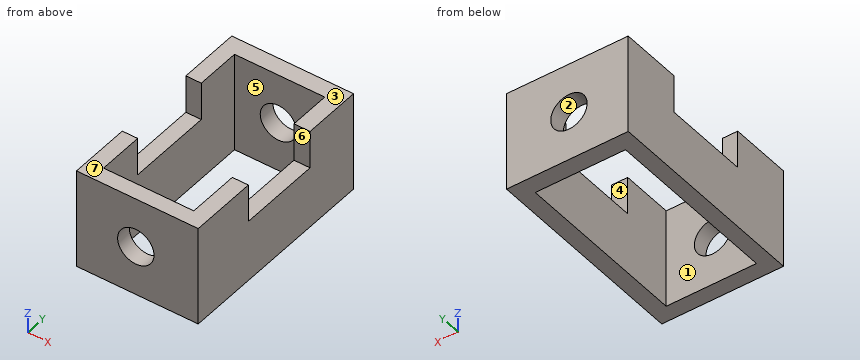
```python
from build123d import *

# Parameters (mm, degrees)
F0_W     = 62.4194853008
F0_H     = 107.7802851796
F0_W_2   = 46.2748277932
F0_H_2   = 90.9063592553
F1_DEPTH = 51.308
F2_W     = 8.2461107522
F2_H     = 42.7914112806
F2_W_2   = 7.8985467553
F2_H_2   = 44.1445242614
F3_DEPTH = 19.558
F4_R     = 9.3280185705
F5_DEPTH = 152.4


with BuildPart() as f1:
    # F0 (on Top) → F1 (new body)
    with BuildSketch(Plane.XY):
        with Locations((-31.2097426504, -8.8457427919)):
            Rectangle(F0_W, F0_H)
        with Locations((-31.3835246488, -9.2003643513)):
            Rectangle(F0_W_2, F0_H_2, mode=Mode.SUBTRACT)
    extrude(amount=F1_DEPTH)

    # F2 (on face) → F3 (cut)
    with BuildSketch(Plane.XY.offset(51.308)):
        with Locations((-4.1230553761, -6.5223816782)):
            Rectangle(F2_W, F2_H)
        with Locations((-58.4702119231, -8.8798655197)):
            Rectangle(F2_W_2, F2_H_2)
    extrude(amount=-F3_DEPTH, mode=Mode.SUBTRACT)

    # F4 (on face) → F5 (cut)
    with BuildSketch(Plane(origin=(0, 45.0443997979, 0), x_dir=(-1, 0, 0), z_dir=(0, 1, 0))):
        with Locations((32.0103727281, 25.654)):
            Circle(F4_R)
    extrude(amount=-F5_DEPTH, mode=Mode.SUBTRACT)


solid = f1.part
```
Can you work these out from the model? Positions are in its coordinate system, mm. Face numbers are marked on the shaded views. A direction names the side the tool comes from. Coordinates: 2 decimals unless noted, no trailing zeros. Loops run counter-clockwise (first coordinate to the right, second up) from the corner with the lowest first, then second, coordinate; pieces in that order, holes last. Notation, with made-up numbers: (27, 60.5) - (84, 60.5) arc R19 cw to (84, 64.5) - close; hole circle Ø3 at (72.5, 76.5). An arc over 180 degrees is marked (long way). Use a Markdown table: item, result.
Item 1: For the marked faces 4, 5, 6 and 7, which set-ups out of +Z, -Z, +X, -X, +Y, -Y let a thin tool reach every point of the face, with its end or its side?
Numbers:
| item | result |
|---|---|
| face 4 | +Z, +X, -X |
| face 5 | +Z, -Z |
| face 6 | +Z, +X |
| face 7 | +Z, +X, -X, +Y, -Y |
Item 2: I want a section at D-D on x = -19. Please give me the cut outline in (y, z), and give its area (3 significant figures).
Numbers:
| item | result |
|---|---|
| outline | (-62.74, 0) - (-54.65, 0) - (-54.65, 51.31) - (-62.74, 51.31) - close; (36.25, 0) - (45.04, 0) - (45.04, 51.31) - (36.25, 51.31) - close |
| area | 866 mm2 |
Item 3: I want a section at B-B on y = -23. Please give me the cut outline in (x, z).
Numbers:
| item | result |
|---|---|
| outline | (-62.42, 0) - (-54.52, 0) - (-54.52, 31.75) - (-62.42, 31.75) - close; (-8.25, 0) - (0, 0) - (0, 31.75) - (-8.25, 31.75) - close |
Item 4: I want a section at A-A on x = -32. Please give me the cut outline in (y, z), and give its area (3 significant figures).
Numbers:
| item | result |
|---|---|
| outline | (-62.74, 0) - (-54.65, 0) - (-54.65, 16.33) - (-62.74, 16.33) - close; (-62.74, 34.98) - (-54.65, 34.98) - (-54.65, 51.31) - (-62.74, 51.31) - close; (36.25, 0) - (45.04, 0) - (45.04, 16.33) - (36.25, 16.33) - close; (36.25, 34.98) - (45.04, 34.98) - (45.04, 51.31) - (36.25, 51.31) - close |
| area | 551 mm2 |
Item 5: If I drill on probe 1 along Y at (x, z) = (-49, 15); probe 2 along X at (y, z) = (-42.5, 15.5); probe 3 along Z at (x, y) = (-36.5, 38), over which ranges is the centre line in solid material (lowest first)? Write a range as from..to.
Numbers:
| item | result |
|---|---|
| probe 1 | y = -62.74..-54.65, 36.25..45.04 |
| probe 2 | x = -62.42..-54.52, -8.25..0 |
| probe 3 | z = 0..17.48, 33.83..51.31 |
Item 6: I want a section at C-C on z = 3. Please give me the cut outline in (x, y).
Numbers:
| item | result |
|---|---|
| outline | (-62.42, -62.74) - (0, -62.74) - (0, 45.04) - (-62.42, 45.04) - close; hole (-54.52, -54.65) - (-8.25, -54.65) - (-8.25, 36.25) - (-54.52, 36.25) - close |
Item 7: Will this pin go through, and if not, where does the flat tip stop? pin 1 (9 mm diameter, centred on x = -3.5, y = -10, fed in from +Z).
Numbers:
| item | result |
|---|---|
| pin 1 | stops at z = 31.75 |
Item 8: We'd pull the mould along Z, two halves only. Please class the marked faces 1, 2 and 3: released by +Z, released by -Z, zero draft, split by the parting line, or undercut.
Numbers:
| item | result |
|---|---|
| face 1 | zero draft |
| face 2 | undercut |
| face 3 | released by +Z |
